```python
from build123d import *

# Parameters (mm, degrees)
SKETCH1_W             = 6
SKETCH1_H             = 12
EXTRUDE1_DEPTH        = 8
SKETCH3_W             = 4
SKETCH3_H             = 8.6
EXTRUDE2_DEPTH        = 1
SKETCH2_R             = 1.25
EXTRUDE3_DEPTH        = 6
EXTRUDE4_DEPTH        = 4
SKETCH6_R             = 5.25
EXTRUDE5_DEPTH        = 1
SKETCH7_R             = 1.25
EXTRUDE6_DEPTH        = 4
CIRPATTERN1_COUNT     = 3
SKETCH8_R             = 2
EXTRUDE7_DEPTH        = 3
FILLET1_R             = 4
M3_TAPPED_HOLE1_D     = 2.5
M3_TAPPED_HOLE1_DEPTH = 6
M3_TAPPED_HOLE1_TIP   = 0.751075774


with BuildPart() as part:
    # Sketch1 → Extrude1 (new body)
    with BuildSketch(Plane.XY):
        with Locations((-1, 0)):
            Rectangle(SKETCH1_W, SKETCH1_H)
    extrude(amount=EXTRUDE1_DEPTH)

    # Sketch3 → Extrude2 (add)
    with BuildSketch(Plane.XY.offset(8)):
        Rectangle(SKETCH3_W, SKETCH3_H)
    extrude(amount=EXTRUDE2_DEPTH)

    # Sketch2 → Extrude3 (cut)
    with BuildSketch(Plane(origin=(0, 0, 0), x_dir=(-1, 0, 0), z_dir=(0, 0, -1))):
        with Locations((1, 3)):
            Circle(SKETCH2_R)
        with Locations((1, -3)):
            Circle(SKETCH2_R)
    extrude(amount=-EXTRUDE3_DEPTH, mode=Mode.SUBTRACT)

    # Sketch4 → Extrude4 (add)
    with BuildSketch(Plane(origin=(2, 0, 0), x_dir=(0, 0, -1), z_dir=(1, 0, 0))):
        with BuildLine():
            Line((-9.900455543, 6), (-8, 6))
            Line((-8, 6), (-8, -6))
            Line((-8, -6), (-9.900455543, -6))
            ThreePointArc((-9.900455543, -6), (-30.12, 0), (-9.900455543, 6))
        make_face()
    extrude(amount=-EXTRUDE4_DEPTH)

    # Sketch6 → Extrude5 (cut)
    with BuildSketch(Plane.ZY.offset(2)):
        with Locations(Location((19.12, 0, 0), (0, 0, 270))):
            Circle(SKETCH6_R)
    extrude(amount=-EXTRUDE5_DEPTH, mode=Mode.SUBTRACT)

    # Sketch7 → Extrude6 (cut)
    with BuildSketch(Plane.ZY.offset(2)):
        with Locations(Location((19.12, -8.5, 0), (0, 0, 270))):
            Circle(SKETCH7_R)
    extrude6 = extrude(amount=-EXTRUDE6_DEPTH, mode=Mode.SUBTRACT)

    # CirPattern1: Extrude6 ×3 about axis
    cirpattern1_axis = Axis((0, 0, 19.12), (1, 0, 0))
    for i in range(1, CIRPATTERN1_COUNT):
        add(extrude6.rotate(cirpattern1_axis, i * 360 / CIRPATTERN1_COUNT), mode=Mode.SUBTRACT)

    # Sketch8 → Extrude7 (cut)
    with BuildSketch(Plane.ZY.offset(1)):
        with Locations(Location((19.12, 0, 0), (0, 0, 270))):
            Circle(SKETCH8_R)
    extrude(amount=-EXTRUDE7_DEPTH, mode=Mode.SUBTRACT)

    # Fillet1
    # the kernel refuses this fillet: 4 mm, written as the material it adds along each edge
    with BuildSketch(Plane(origin=(2, 6, 9.900455543), x_dir=(0, 0, -1), z_dir=(-1, 0, 0))) as fillet1_piece_1_section:
        with BuildLine():
            CenterArc((1.96079543, -4), FILLET1_R, 90, 48.189685104)
            ThreePointArc((-1.02062854, -1.333333333), (-0.484835824, -0.686169688), (0, 0))
            Line((0, 0), (1.96079543, 0))
        make_face()
    fillet1_piece_1 = extrude(amount=4, mode=Mode.PRIVATE)
    fillet1_piece_1 = split(fillet1_piece_1, bisect_by=Plane(origin=(0, 5.96007597, 8), z_dir=(0, 0, -1)), keep=Keep.TOP, mode=Mode.PRIVATE)
    add(fillet1_piece_1)
    with BuildSketch(Plane(origin=(2, 6, 9.900455543), x_dir=(0, 0, -1), z_dir=(-1, 0, 0))) as fillet1_piece_2_section:
        with BuildLine():
            CenterArc((1.96079543, -4), FILLET1_R, 90, 48.189685104)
            ThreePointArc((-1.02062854, -1.333333333), (-0.484835824, -0.686169688), (0, 0))
            Line((0, 0), (1.96079543, 0))
        make_face()
    fillet1_piece_2 = extrude(amount=4, mode=Mode.PRIVATE)
    fillet1_piece_2 = split(fillet1_piece_2, bisect_by=Plane(origin=(0, 6.284176822, 8), z_dir=(0, 0, 1)), keep=Keep.TOP, mode=Mode.PRIVATE)
    add(fillet1_piece_2)
    with BuildSketch(Plane(origin=(2, 6, 9.900455543), x_dir=(0, 0, -1), z_dir=(-1, 0, 0))) as fillet1_piece_3_section:
        with BuildLine():
            CenterArc((1.96079543, -4), FILLET1_R, 90, 48.189685104)
            ThreePointArc((-1.02062854, -1.333333333), (-0.484835824, -0.686169688), (0, 0))
            Line((0, 0), (1.96079543, 0))
        make_face()
    fillet1_piece_3 = extrude(amount=8.901988576, mode=Mode.PRIVATE)
    fillet1_piece_3 = split(fillet1_piece_3, bisect_by=Plane(origin=(-4, 5.96007597, 7.969858609), z_dir=(1, 0, 0)), keep=Keep.TOP, mode=Mode.PRIVATE)
    fillet1_piece_3 = split(fillet1_piece_3, bisect_by=Plane(origin=(-3, 5.96007597, 8), z_dir=(0, 0, -1)), keep=Keep.TOP, mode=Mode.PRIVATE)
    fillet1_piece_3 = split(fillet1_piece_3, bisect_by=Plane(origin=(-2, 5.96007597, 7.969858609), z_dir=(-1, 0, 0)), keep=Keep.TOP, mode=Mode.PRIVATE)
    add(fillet1_piece_3)
    with BuildSketch(Plane(origin=(2, -6, 9.900455543), x_dir=(0, -0.794064421171895, 0.6078336080120474), z_dir=(-1, 0, 0))) as fillet1_piece_4_section:
        with BuildLine():
            CenterArc((1.984420324, -3.98833232), FILLET1_R, 94.377291872, 48.189685104)
            Line((-1.191837361, -1.556997888), (0, 0))
            ThreePointArc((0, 0), (0.839562445, -0.032086119), (1.679124889, 0))
        make_face()
    fillet1_piece_4 = extrude(amount=4, mode=Mode.PRIVATE)
    fillet1_piece_4 = split(fillet1_piece_4, bisect_by=Plane(origin=(0, -6.284176822, 8), z_dir=(0, 0, 1)), keep=Keep.TOP, mode=Mode.PRIVATE)
    add(fillet1_piece_4)
    with BuildSketch(Plane(origin=(2, -6, 9.900455543), x_dir=(0, -0.794064421171895, 0.6078336080120474), z_dir=(-1, 0, 0))) as fillet1_piece_5_section:
        with BuildLine():
            CenterArc((1.984420324, -3.98833232), FILLET1_R, 94.377291872, 48.189685104)
            Line((-1.191837361, -1.556997888), (0, 0))
            ThreePointArc((0, 0), (0.839562445, -0.032086119), (1.679124889, 0))
        make_face()
    fillet1_piece_5 = extrude(amount=4, mode=Mode.PRIVATE)
    fillet1_piece_5 = split(fillet1_piece_5, bisect_by=Plane(origin=(0, -5.96007597, 8), z_dir=(0, 0, -1)), keep=Keep.TOP, mode=Mode.PRIVATE)
    add(fillet1_piece_5)
    with BuildSketch(Plane(origin=(2, -6, 9.900455543), x_dir=(0, -0.794064421171895, 0.6078336080120474), z_dir=(-1, 0, 0))) as fillet1_piece_6_section:
        with BuildLine():
            CenterArc((1.984420324, -3.98833232), FILLET1_R, 94.377291872, 48.189685104)
            Line((-1.191837361, -1.556997888), (0, 0))
            ThreePointArc((0, 0), (0.839562445, -0.032086119), (1.679124889, 0))
        make_face()
    fillet1_piece_6 = extrude(amount=8.901988576, mode=Mode.PRIVATE)
    fillet1_piece_6 = split(fillet1_piece_6, bisect_by=Plane(origin=(-4, -5.96007597, 7.969858609), z_dir=(1, 0, 0)), keep=Keep.TOP, mode=Mode.PRIVATE)
    fillet1_piece_6 = split(fillet1_piece_6, bisect_by=Plane(origin=(-3, -5.96007597, 8), z_dir=(0, 0, -1)), keep=Keep.TOP, mode=Mode.PRIVATE)
    fillet1_piece_6 = split(fillet1_piece_6, bisect_by=Plane(origin=(-2, -5.96007597, 7.969858609), z_dir=(-1, 0, 0)), keep=Keep.TOP, mode=Mode.PRIVATE)
    add(fillet1_piece_6)

    # M3 Tapped Hole1
    with Locations(Plane(origin=(-1, 3, 0), x_dir=(-1, 0, 0), z_dir=(0, 0, -1))):
        with Locations((0, 0), (0, -6)):
            Hole(M3_TAPPED_HOLE1_D / 2, depth=M3_TAPPED_HOLE1_DEPTH)
            with Locations((0, 0, -(M3_TAPPED_HOLE1_DEPTH + M3_TAPPED_HOLE1_TIP / 2))):  # 118° drill point
                Cone(0, M3_TAPPED_HOLE1_D / 2, M3_TAPPED_HOLE1_TIP, mode=Mode.SUBTRACT)


solid = part.part
```
Geometry check sheet. Reference: the model listing, model coordinates, mm. A direction names the side the tool comes from. Give positions to 0.01 mm unless a question says otherwise; leave off trailing zeros. Order: outer loops, then holes, each group sorted by start corner. A loop starts at its lowest first (then second) coordinate and runs counter-clockwise, first axis right, second up.
1. Section check C-C, the plane x = 0.8. Enter the section's corners in (y, z) (3 decimals).
2. Section check A-A, the plane y = 0. Enter the section's corners in (x, z).
3. Access from +Z, -Z, +X, -X, +Y, -Y to the whole of each face (thin tool, end or side, straight path). Record for faces 1 (the face through (-0.079, 3.845, 2.958)), 2 (the face through (-1, -2.3, 19.2)), 3 (the face through (-1, 6, 4)).
4. Gauge pin test, flat ends, axial feed: pin 1 Ø2 at (y, z) = (-1, 23) entering from -X; pin 2 Ø2 at (x, y) = (-2, -3.5) entering from +Z; pin 3 Ø3 at (x, y) = (-1, -3) entering from +Z; pin 4 Ø3 at (x, y) = (-1, 3) entering from -Z. Record the tip position at first contact, or that the pin passes through.
5. Thickness scan on L1, parallel to Y at x = -1, z = 4.1; L2, parallel to X at y = -3, z = 3; L3, parallel to Z at x = -3.7, y = -1. Record the ranges inside material, lowest first.
6. Section check B-B, the plane z = 19.12. Enter the section's corners in (x, y).
7. Release check for a two-part mould opening along Z. For faces 4 (the face through (-1.21, -2.93, 6.62)), 5 (the face through (0.479, -1.075, 20.806)), 6 (the face through (-4, 0, 4)), 7 (the face through (-0.03, 4.52, 10.54)) record: pulls with the +Z half, pulls with the -Z half, needs draft (parallel to the pull), parting line crosses it, or undercut.
8. Section check D-D, the plane z = 12. Enter the section's corners in (x, y).
Values follow:
1. outline: (-7.333, 10.921) arc R4 cw to (-6, 7.94) - (-6, 0) - (6, 0) - (6, 7.94) arc R4 cw to (7.333, 10.921) arc R11 ccw (long way) to start; hole circle Ø2.5 at (-8.5, 19.12); hole circle Ø4 at (0, 19.12); hole circle Ø2.5 at (4.25, 11.759); hole circle Ø2.5 at (4.25, 26.481)
2. outline: (-4, 0) - (2, 0) - (2, 17.12) - (-1, 17.12) - (-1, 13.87) - (-2, 13.87) - (-2, 8) - (-4, 8) - close; (-2, 24.37) - (-1, 24.37) - (-1, 21.12) - (2, 21.12) - (2, 30.12) - (-2, 30.12) - close
3. face 1: -Z
3. face 2: -X
3. face 3: -Z, +X, -X, +Y
4. pin 1: stops at x = -1
4. pin 2: stops at z = 29.83
4. pin 3: stops at z = 30.02
4. pin 4: stops at z = 0
5. L1: y = -6 to -4.25, -1.75 to 1.75, 4.25 to 6
5. L2: x = -4 to -2.25, 0.25 to 2
5. L3: z = 0 to 8
6. outline: (-2, -11) - (2, -11) - (2, -9.75) - (-2, -9.75) - close; (-2, -7.25) - (2, -7.25) - (2, -2) - (-1, -2) - (-1, -5.25) - (-2, -5.25) - close; (-2, 5.25) - (-1, 5.25) - (-1, 2) - (2, 2) - (2, 11) - (-2, 11) - close
7. face 4: pulls with the -Z half
7. face 5: undercut
7. face 6: needs draft
7. face 7: undercut
8. outline: (-2, -8.38) - (2, -8.38) - (2, 3.02) - (-2, 3.02) - close; (-2, 5.48) - (2, 5.48) - (2, 8.38) - (-2, 8.38) - close
